from build123d import *

# Parameters (mm, degrees)
SKETCH1_W           = 177.8
SKETCH1_H           = 101.6
BOSS_EXTRUDE1_DEPTH = 19.05
CUT_EXTRUDE1_DEPTH  = 39.1
SKETCH3_R           = 3.175
SKETCH3_R_2         = 6.35
SKETCH3_R_3         = 15.0495
CUT_EXTRUDE2_DEPTH  = 102.6


with BuildPart() as part:
    # Sketch1 → Boss-Extrude1 (new body, symmetric)
    with BuildSketch(Plane(origin=(0, 0, 0), x_dir=(1, 0, 0), z_dir=(0, 1, 0))):
        Rectangle(SKETCH1_W, SKETCH1_H)
    extrude(amount=BOSS_EXTRUDE1_DEPTH, both=True)

    # Sketch2 → Cut-Extrude1 (cut, through all)
    with BuildSketch(Plane(origin=(0, 19.05, 0), x_dir=(1, 0, 0), z_dir=(0, 1, 0))):
        Polygon((-79.375, 24.765), (-69.215, 34.925), (-45.085, 34.925), (-34.925, 24.765), (-34.925, -24.765), (-45.085, -34.925), (-69.215, -34.925), (-79.375, -24.765), align=None)
        with BuildLine():
            Line((-12.7, 38.1), (12.7, 38.1))
            ThreePointArc((12.7, 38.1), (21.680256121, 34.380256121), (25.4, 25.4))
            Line((25.4, 25.4), (25.4, -25.4))
            ThreePointArc((25.4, -25.4), (21.680256121, -34.380256121), (12.7, -38.1))
            Line((12.7, -38.1), (-12.7, -38.1))
            ThreePointArc((-12.7, -38.1), (-21.680256121, -34.380256121), (-25.4, -25.4))
            Line((-25.4, -25.4), (-25.4, 25.4))
            ThreePointArc((-25.4, 25.4), (-21.680256121, 34.380256121), (-12.7, 38.1))
        make_face()
        Polygon((64.338522628, 6.35), (75.337045256, 25.4), (64.338522628, 44.45), (42.341477372, 44.45), (31.342954744, 25.4), (42.341477372, 6.35), align=None)
        Polygon((42.341477372, -6.35), (64.338522628, -6.35), (75.337045256, -25.4), (64.338522628, -44.45), (42.341477372, -44.45), (31.342954744, -25.4), align=None)
    extrude(amount=-CUT_EXTRUDE1_DEPTH, mode=Mode.SUBTRACT)

    # Sketch3 → Cut-Extrude2 (cut, through all)
    with BuildSketch(Plane.XY.offset(50.8)):
        with Locations((-88.9, 12.7)):
            Circle(SKETCH3_R)
        with Locations((-88.9, 0)):
            Circle(SKETCH3_R_2)
        with Locations((-88.9, -12.7)):
            Circle(SKETCH3_R)
        with Locations((53.34, 0)):
            Circle(SKETCH3_R_3)
        Polygon((-75.565, 6.35), (-69.215, 12.7), (-45.085, 12.7), (-38.735, 6.35), (-38.735, -6.35), (-45.085, -12.7), (-69.215, -12.7), (-75.565, -6.35), align=None)
        Polygon((9.227090106, -12.7), (14.929745408, 4.850968343), (0, 15.698063314), (-14.929745408, 4.850968343), (-9.227090106, -12.7), align=None)
        Polygon((88.9, 9.525), (79.375, 15.024261314), (79.375, -15.024261314), (88.9, -9.525), align=None)
    extrude(amount=-CUT_EXTRUDE2_DEPTH, mode=Mode.SUBTRACT)


solid = part.part
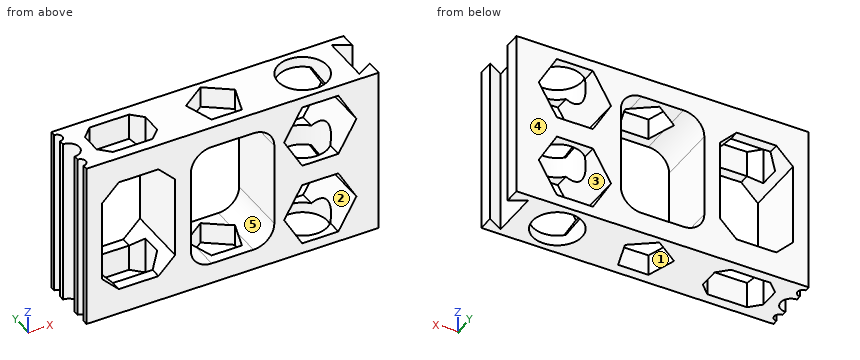
Geometry check sheet. Reference: the model listing, model coordinates, mm. Face numbers are marked on the shaded views. A direction names the side the tool comes from. Round coordinates to 2 decimals unless told otherwise and drop trailing zeros. Order: outer loops, then holes, each group sorted by start corner. A loop starts at its lowest first (then second) coordinate and runs counter-clockwise, first axis right, second up. Notation, with made-up numbers: M 27,80.25 L 72,80.25 A24 cw 72,115.25 Z; hole C 78.5,2.5 d2. An arc over 180 degrees is marked long. Answer in a Markdown table with one row per item.
(1) Go/stop test with flat-tipped pins: P1, Ø1, axis at y = -13, z = -36, coming from the -X side; P2, Ø4, axis at y = 2, z = 39, coming from the +X side (3 decimals). Record where each tip stops, or that it passes through.
Responses:
| item | result |
|---|---|
| P1 | stops at x = -85.83 |
| P2 | stops at x = 79.375 |
(2) Tool access check on the marked faces 1 and 2. Record the directions out of +Z, -Z, +X, -X, +Y, -Y that give a thin tool (end or side, any length) a straight path to the whole face; none if there is none.
Responses:
| item | result |
|---|---|
| face 1 | +Z, -Z |
| face 2 | +Y, -Y |
(3) Draft check along X on the marked faces 3, 4 and 5. Enter one of: released by +X, released by -X, zero draft, split by the parting line, or undercut.
Responses:
| item | result |
|---|---|
| face 3 | undercut |
| face 4 | zero draft |
| face 5 | undercut |
(4) Sectioned sample at A-A, the plane z = 4. State how many separate pieces and enclosed holes the cut face has, and give its area (3 significant figures).
Responses:
| item | result |
|---|---|
| separate pieces | 3 |
| enclosed holes | 1 |
| area | 2,100 mm² |
(5) Sectioned sample at B-B, the plane x = 53.34. Record the cut outline in (y, z).
Responses:
| item | result |
|---|---|
| outline | M -19.05,-50.8 L -15.05,-50.8 L -15.05,-44.45 L -19.05,-44.45 Z; M -19.05,-6.35 L -15.05,-6.35 L -15.05,6.35 L -19.05,6.35 Z; M -19.05,44.45 L -15.05,44.45 L -15.05,50.8 L -19.05,50.8 Z; M 15.05,-50.8 L 19.05,-50.8 L 19.05,-44.45 L 15.05,-44.45 Z; M 15.05,-6.35 L 19.05,-6.35 L 19.05,6.35 L 15.05,6.35 Z; M 15.05,44.45 L 19.05,44.45 L 19.05,50.8 L 15.05,50.8 Z |
(6) Scan lines: probe 1 along Y at (x, z) = (-62.5, -46); probe 2 along Y at (x, z) = (53, -47); probe 3 along X at (y, z) = (-16, -2) (3 decimals). Record each from-to range of solid material in increasing order. Write a range as from..to.
Responses:
| item | result |
|---|---|
| probe 1 | y = -19.05..-12.7, 12.7..19.05 |
| probe 2 | y = -19.05..-15.05, 15.05..19.05 |
| probe 3 | x = -88.9..-79.375, -34.925..-25.4, 25.4..88.9 |
(7) Sectioned sample at C-C, the plane z = 20.5. Record the cut outline in (x, y) (3 decimals), and give its area (3 significant figures).
Responses:
| item | result |
|---|---|
| outline | M -88.9,-19.05 L -79.375,-19.05 L -79.375,19.05 L -88.9,19.05 L -88.9,15.875 A3.175 cw -88.9,9.525 L -88.9,6.35 A6.35 cw -88.9,-6.35 L -88.9,-9.525 A3.175 cw -88.9,-15.875 Z; M -34.925,-19.05 L -25.4,-19.05 L -25.4,19.05 L -34.925,19.05 Z; M 25.4,-19.05 L 34.172,-19.05 L 34.172,19.05 L 25.4,19.05 Z; M 72.508,-19.05 L 88.9,-19.05 L 88.9,-9.525 L 79.375,-15.024 L 79.375,15.024 L 88.9,9.525 L 88.9,19.05 L 72.508,19.05 Z |
| area | 1,360 mm² |
